For this review, take the finished solid that the model builds, in its own axes (mm). Face numbers are marked on the shaded views. Round coordinates to 2 decimals unless told otherwise and drop trailing zeros. Order: outer loops, then holes, each group sorted by start corner. A loop starts at its lowest first (then second) coordinate and runs counter-clockwise, first axis right, second up. Notation, with made-up numbers: M 10.25,1.5 L 48.25,1.5 A20 cw 48.25,7.5 Z; hole C -1.75,48.5 d4. An arc over 180 degrees is marked long. Use a Markdown table: item, result.
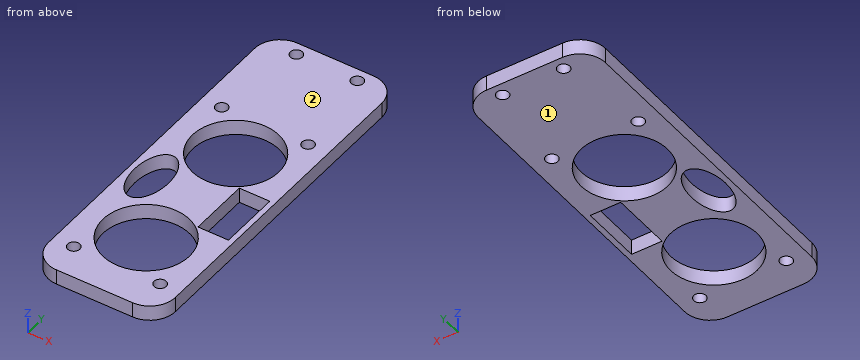
from build123d import *

# Parameters (mm, degrees)
SKETCH1_W            = 25
SKETCH1_H            = 70
SKETCH1_R            = 8.5
SKETCH1_R_2          = 1.2
BOSS_EXTRUDE1_DEPTH  = 3
FILLET1_R            = 5
M2_CLEARANCE_HOLE1_D = 2.4
SKETCH4_W            = 6
SKETCH4_H            = 12
CUT_EXTRUDE1_DEPTH   = 3
SKETCH8_RX           = 6.264875336
SKETCH8_RY           = 3.331610005
CUT_EXTRUDE2_DEPTH   = 3


with BuildPart() as part:
    # Sketch1 → Boss-Extrude1 (new body)
    with BuildSketch(Plane.XY):
        with Locations((12.5, -35)):
            Rectangle(SKETCH1_W, SKETCH1_H)
        with Locations((12.5, -29)):
            Circle(SKETCH1_R, mode=Mode.SUBTRACT)
        with Locations((12.5, -55)):
            Circle(SKETCH1_R, mode=Mode.SUBTRACT)
        with Locations((21, -63.5)):
            Circle(SKETCH1_R_2, mode=Mode.SUBTRACT)
        with Locations((4, -63.5)):
            Circle(SKETCH1_R_2, mode=Mode.SUBTRACT)
        with Locations((4, -20.5)):
            Circle(SKETCH1_R_2, mode=Mode.SUBTRACT)
        with Locations((21, -20.5)):
            Circle(SKETCH1_R_2, mode=Mode.SUBTRACT)
    extrude(amount=BOSS_EXTRUDE1_DEPTH)

    # Fillet1
    fillet1_edges = [part.edges().sort_by_distance(p)[0] for p in [
        (0, 0, 1.5),
        (25, 0, 1.5),
        (25, -70, 1.5),
        (0, -70, 1.5),
    ]]
    fillet(fillet1_edges, radius=FILLET1_R)

    # M2 Clearance Hole1 (through all)
    with Locations(Plane.XY.offset(3)):
        with Locations((6.5, -2.5), (18.5, -2.5)):
            Hole(M2_CLEARANCE_HOLE1_D / 2)

    # Sketch4 → Cut-Extrude1 (cut)
    with BuildSketch(Plane.XY.offset(3)):
        with Locations((20.953787987, -42)):
            Rectangle(SKETCH4_W, SKETCH4_H)
    extrude(amount=-CUT_EXTRUDE1_DEPTH, mode=Mode.SUBTRACT)

    # Sketch8 → Cut-Extrude2 (cut)
    with BuildSketch(Plane(origin=(0, 0, 0), x_dir=(-1, 0, 0), z_dir=(0, 0, -1))):
        with Locations(Location((-4.382036581, -41.5), (0, 0, -90))):
            Ellipse(SKETCH8_RX, SKETCH8_RY)
    extrude(amount=-CUT_EXTRUDE2_DEPTH, mode=Mode.SUBTRACT)


solid = part.part
Q1. Wall thickness on line 1 along Y through (x, z) = (12.5, 0.65); line 2 along X through (y, z) = (-33, 0.45); line 3 along Y through (x, z) = (16.25, 1.1): over which ranges is each line inside the solid? List them lowest first. Write a range as [from, to].
Determined:
| item | result |
|---|---|
| line 1 | y = [-70, -63.5], [-46.5, -37.5], [-20.5, 0] |
| line 2 | x = [0, 5], [20, 25] |
| line 3 | y = [-70, -62.63], [-47.37, -36.63], [-21.37, 0] |
Q2. Draft analysis for pull direction Z (two halves, no side actions). For the marked faces 1 and 2, state which applies: pulls with the +Z half, pulls with the -Z half, needs draft (parallel to the pull), parting line crosses it, or undercut.
Determined:
| item | result |
|---|---|
| face 1 | pulls with the -Z half |
| face 2 | pulls with the +Z half |
Q3. Add section B-B (y = -29). Write out the cut boundary in (x, z), then the cut area to 3 significant figures.
Determined:
| item | result |
|---|---|
| outline | M 0,0 L 4,0 L 4,3 L 0,3 Z; M 21,0 L 25,0 L 25,3 L 21,3 Z |
| area | 24.0 mm^2 |
Q4. Clearance check with flat-ended pins moving along their axes: pin 1 (0.9 mm diameter, centred on x = 21.5, z = 2, fed in from -Y); pin 2 (1.9 mm diameter, centred on x = 21, y = -63.5, fed in from -Z). State where each tip first meets the part, or that it passes through.
Determined:
| item | result |
|---|---|
| pin 1 | stops at y = -69.89 |
| pin 2 | passes through |
Q5. Add section C-C (x = 6.25). Give the number of separate pieces and of enclosed holes in the cut face, then the cut area to 3 significant figures.
Determined:
| item | result |
|---|---|
| separate pieces | 5 |
| enclosed holes | 0 |
| area | 103 mm^2 |
Q6. Add section A-A (x = 12.5). Write out the cut boundary in (y, z), then the cut area to 3 significant figures.
Determined:
| item | result |
|---|---|
| outline | M -70,0 L -63.5,0 L -63.5,3 L -70,3 Z; M -46.5,0 L -37.5,0 L -37.5,3 L -46.5,3 Z; M -20.5,0 L 0,0 L 0,3 L -20.5,3 Z |
| area | 108 mm^2 |
